```python
from build123d import *

# Parameters (mm, degrees)
SKETCH_1_W          = 80
SKETCH_1_H          = 80
EXTRUDE_1_DEPTH     = 3
SKETCH_2_R          = 4.05
CUT_EXTRUDE_1_DEPTH = 3
SKETCH_3_R          = 2.7
CUT_EXTRUDE_2_DEPTH = 3


with BuildPart() as part:
    # 草图1 → 凸台-拉伸1 (new body)
    with BuildSketch(Plane(origin=(0, 0, 0), x_dir=(1, 0, 0), z_dir=(0, 1, 0))):
        Rectangle(SKETCH_1_W, SKETCH_1_H)
    extrude(amount=EXTRUDE_1_DEPTH)

    # 草图2 → 切除-拉伸1 (cut)
    with BuildSketch(Plane(origin=(0, 3, 0), x_dir=(1, 0, 0), z_dir=(0, 1, 0))):
        with Locations(Location((0, 0, 0), (0, 0, 270))):
            Circle(SKETCH_2_R)
    extrude(amount=-CUT_EXTRUDE_1_DEPTH, mode=Mode.SUBTRACT)

    # 草图3 → 切除-拉伸2 (cut)
    with BuildSketch(Plane(origin=(0, 3, 0), x_dir=(1, 0, 0), z_dir=(0, 1, 0))):
        with Locations(Location((16.125, 0, 0), (0, 0, 270))):
            Circle(SKETCH_3_R)
        with Locations(Location((-16.125, 0, 0), (0, 0, 270))):
            Circle(SKETCH_3_R)
    extrude(amount=-CUT_EXTRUDE_2_DEPTH, mode=Mode.SUBTRACT)


solid = part.part
```
Read the model definition and answer for the solid it produces. Units are mm, in the model's axes. Coordinates: 2 decimals unless noted, no trailing zeros. Loops run counter-clockwise (first coordinate to the right, second up) from the corner with the lowest first, then second, coordinate; pieces in that order, holes last.
(1) Consider line 1 along X through (y, z) = (1.55, 0) (3 decimals); line 2 along X through (y, z) = (0.7, 0.5); line 3 along Z through (x, y) = (3.5, 0.2). Determine where each line is inside the solid, lowest interval first.
Solution:
line 1: x = -40 to -18.825, -13.425 to -4.05, 4.05 to 13.425, 18.825 to 40
line 2: x = -40 to -18.78, -13.47 to -4.02, 4.02 to 13.47, 18.78 to 40
line 3: z = -40 to -2.04, 2.04 to 40
(2) The mould has two halves that part along Z. Classify faces 1 (the face through (-13.448, 1.521, -0.351)), 2 (the face through (8, 0, -1)), 3 (the face through (-1, 1, 40)), 4 (the face through (-3.593, 1.521, 1.869)): released by +Z, released by -Z, zero draft, split by the parting line, or undercut.
Solution:
face 1: undercut
face 2: zero draft
face 3: released by +Z
face 4: undercut
(3) A flat-ended cylindrical pin translates along its axis: pin 1 Ø5 at (x, z) = (16.125, 0) entering from +Y. Find the tip coordinate at first contact, or state that the pin passes through.
Solution:
pin 1: passes through
(4) The part is cut by section A-A (x = 0). Determine the outline of the cut face in (y, z).
Solution:
outline: (0, -40) - (3, -40) - (3, -4.05) - (0, -4.05) - close; (0, 4.05) - (3, 4.05) - (3, 40) - (0, 40) - close
(5) The part is cut by section C-C (y = 2). Determine the outline of the cut face in (x, z) (3 decimals), and give its area (3 significant figures).
Solution:
outline: (-40, -40) - (40, -40) - (40, 40) - (-40, 40) - close; hole circle Ø5.4 at (-16.125, 0); hole circle Ø8.1 at (0, 0); hole circle Ø5.4 at (16.125, 0)
area: 6,300 mm2
(6) The part is cut by section B-B (z = 0). Determine the outline of the cut face in (x, y) (3 decimals).
Solution:
outline: (-40, 0) - (-18.825, 0) - (-18.825, 3) - (-40, 3) - close; (-13.425, 0) - (-4.05, 0) - (-4.05, 3) - (-13.425, 3) - close; (4.05, 0) - (13.425, 0) - (13.425, 3) - (4.05, 3) - close; (18.825, 0) - (40, 0) - (40, 3) - (18.825, 3) - close
